Input: dimensioned drawing with shaded views. Units: mm. Origin: part minimum x, y, z. A direction names the side the tool comes from. Give positions to 0.01 mm unless a question says otherwise; leave off trailing zeros. Write each loop counter-clockwise with the first axis right and the second up, starting at its lowest first coordinate (ties: lowest second). Pieces come first, ordered by that corner, then holes. Notation, with made-up numbers: (-38, 57) -> (-31, 57) arc R21 cw to (-31, 80) -> close; hole circle Ø5 at (68.25, -31). An arc over 180 degrees is marked (long way). Answer as a JSON object with one key per item and string values. Group by question number.
(1) Set-up query: the marked faces 1, 2 and 3. Return all of +Z, -Z, +X, -X, +Y, -Y with unobstructed straight access to the full face (end or side cutting, diameter ignored); none if empty.
(2) Section query D-D on z = 1.5. Output: boundary loops of the cut face in (x, y), plus the area to 3 significant figures.
(3) Material intervals for probe 1 along Z at (x, y) = (15, 18.25); probe 2 along Z at (x, y) = (15.75, 3.25); probe 3 along X at (y, z) = (15, 22.25), sorted ascending.
(4) Section query B-B on x = 2. Output: boundary loops of the cut face in (y, z), plus the area to 3 significant figures.
(5) Section query A-A on y = 15. Output: boundary loops of the cut face in (x, z), plus the area to 3 significant figures.
(6) Section query C-C on x = 22. Output: boundary loops of the cut face in (y, z).
(7) Contact query for flat-ended pins moving along their axis: pin 1 Ø8 at (y, z) = (11, 20.5) entering from -X; pin 2 Ø3 at (x, z) = (17.5, 14) entering from -Y; pin 3 Ø5 at (x, z) = (15, 10) entering from +Y. Output: stop coordinate, or through.
(8) Draft query along X for the marked faces 4, 5 and 6. Return one class per face: +X half, -X half, draft (parallel to the pull), parting line (faces both ways), or undercut.
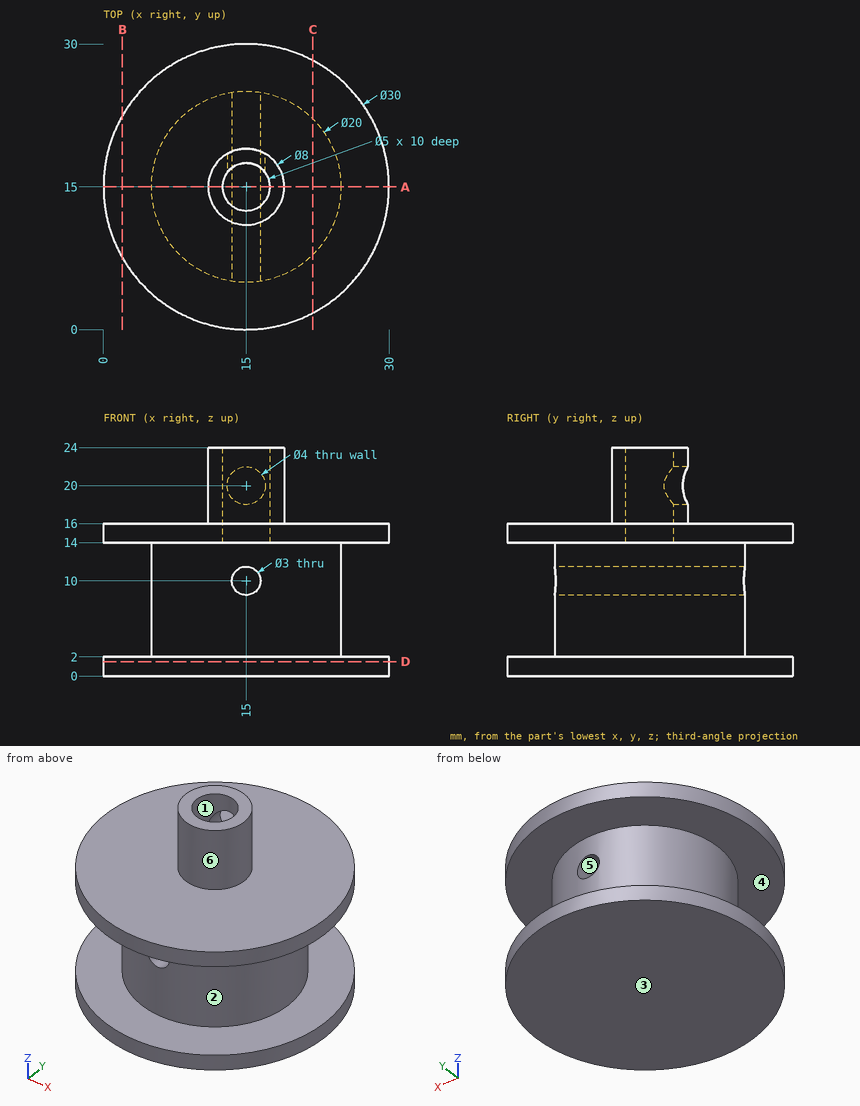
Answer list:
{
 "1": {"face 1": "+Z", "face 2": "none", "face 3": "-Z, +X, -X, +Y, -Y"},
 "2": {"outline": "circle Ø30 at (15, 15)", "area": "707 mm2"},
 "3": {"probe 1": "0 to 8.5, 11.5 to 18, 22 to 24", "probe 2": "0 to 2, 14 to 16", "probe 3": "11 to 12.5, 17.5 to 19"},
 "4": {"outline": "(7.52, 0) -> (22.48, 0) -> (22.48, 2) -> (7.52, 2) -> close; (7.52, 14) -> (22.48, 14) -> (22.48, 16) -> (7.52, 16) -> close", "area": "59.9 mm2"},
 "5": {"outline": "(0, 0) -> (30, 0) -> (30, 2) -> (25, 2) -> (25, 14) -> (30, 14) -> (30, 16) -> (19, 16) -> (19, 24) -> (17.5, 24) -> (17.5, 14) -> (12.5, 14) -> (12.5, 24) -> (11, 24) -> (11, 16) -> (0, 16) -> (0, 14) -> (5, 14) -> (5, 2) -> (0, 2) -> close; hole circle Ø3 at (15, 10)", "area": "367 mm2"},
 "6": {"outline": "(1.73, 0) -> (28.27, 0) -> (28.27, 2) -> (22.14, 2) -> (22.14, 14) -> (28.27, 14) -> (28.27, 16) -> (1.73, 16) -> (1.73, 14) -> (7.86, 14) -> (7.86, 2) -> (1.73, 2) -> close"},
 "7": {"pin 1": "x = 11", "pin 2": "y = 0.03", "pin 3": "y = 25"},
 "8": {"face 4": "draft", "face 5": "undercut", "face 6": "parting line"}
}
